from build123d import *

# Parameters (mm, degrees)
BOSS_EXTRUDE1_DEPTH = 6.35


with BuildPart() as part:
    # Sketch3 → Boss-Extrude1 (new body)
    with BuildSketch(Plane.XY):
        Polygon((25.54605, 133.35), (5.9944, 133.35), (5.9944, 99.26955), (0, 99.26955), (0, 77.53985), (5.9944, 77.53985), (5.9944, 55.81015), (0, 55.81015), (0, 34.08045), (5.9944, 34.08045), (5.9944, 12.35075), (5.9944, 0), (25.54605, 0), (25.54605, 5.9944), (47.27575, 5.9944), (47.27575, 0), (69.00545, 0), (69.00545, 5.9944), (90.73515, 5.9944), (90.73515, 0), (112.46485, 0), (112.46485, 5.9944), (134.19455, 5.9944), (134.19455, 0), (155.92425, 0), (155.92425, 5.9944), (177.65395, 5.9944), (177.65395, 0), (197.2056, 0), (197.2056, 34.08045), (203.2, 34.08045), (203.2, 55.81015), (197.2056, 55.81015), (197.2056, 77.53985), (203.2, 77.53985), (203.2, 99.26955), (197.2056, 99.26955), (197.2056, 120.99925), (197.2056, 133.35), (177.65395, 133.35), (177.65395, 127.3556), (155.92425, 127.3556), (155.92425, 133.35), (134.19455, 133.35), (134.19455, 127.3556), (112.46485, 127.3556), (112.46485, 133.35), (90.73515, 133.35), (90.73515, 127.3556), (69.00545, 127.3556), (69.00545, 133.35), (47.27575, 133.35), (47.27575, 127.3556), (25.54605, 127.3556), align=None)
    extrude(amount=BOSS_EXTRUDE1_DEPTH)


solid = part.part
Model file for the job. Use its own axes, mm. A direction names the side the tool comes from. Give positions to 0.01 mm unless a question says otherwise; leave off trailing zeros. Write each loop counter-clockwise with the first axis right and the second up, starting at its lowest first coordinate (ties: lowest second). Pieces come first, ordered by that corner, then holes. Notation, with made-up numbers: (-10.75, 61.25) -> (-2.75, 61.25) arc R10 cw to (-2.75, 74.25) -> close; hole circle Ø6 at (-12, 9.25). An arc over 180 degrees is marked (long way). Write item = value, one per line.
(1) Mould opens along Y. For faces 1 (the face through (197.206, 67, 3)), 2 (the face through (134.195, 130, 3)), 3 (the face through (123, 127.356, 3)) say: released by +Y, released by -Y, zero draft, split by the parting line, or undercut.
Determined:
face_1 = undercut
face_2 = zero draft
face_3 = released by +Y
(2) Probe line 1 along Y through (x, z) = (116.5, 1); line 2 along X through (y, z) = (105, 6.25). List the from-to ranges inside material, lowest first.
Determined:
line_1 = 5.99 to 127.36
line_2 = 5.99 to 197.21
(3) Flat gauge pins, fed straight in: P1, Ø1.5, axis at y = 105.5, z = 2, coming from the -X side; P2, Ø4, axis at x = 44, y = 119, coming from the -Z side; P3, Ø3, axis at y = 129.5, z = 3.5, coming from the +X side; P4, Ø3, axis at x = 33.5, z = 3.5, coming from the +Y side. Where does each tip first touch, or does it go through?
Determined:
P1 = 5.99
P2 = 0
P3 = 197.21
P4 = 127.36
(4) Slice it at A-A, the plane y = 108. Give the cut face in (x, z).
Determined:
outline = (5.99, 0) -> (197.21, 0) -> (197.21, 6.35) -> (5.99, 6.35) -> close
(5) Slice it at B-B, the plane x = 127. Give the cut face in (y, z), then the cut area to 3 significant figures.
Determined:
outline = (5.99, 0) -> (127.36, 0) -> (127.36, 6.35) -> (5.99, 6.35) -> close
area = 771 mm2
(6) Tool access for faces 4 (the face through (134.195, 3, 3)), 5 (the face through (177.654, 130, 3)), 6 (the face through (197.206, 17, 3)): list every direction of +Z, -Z, +X, -X, +Y, -Y with a clear straight run to the whole face (end or side of a thin tool).
Determined:
face_4 = +Z, -Z, -Y
face_5 = +Z, -Z, +Y
face_6 = +Z, -Z, +X, -Y
